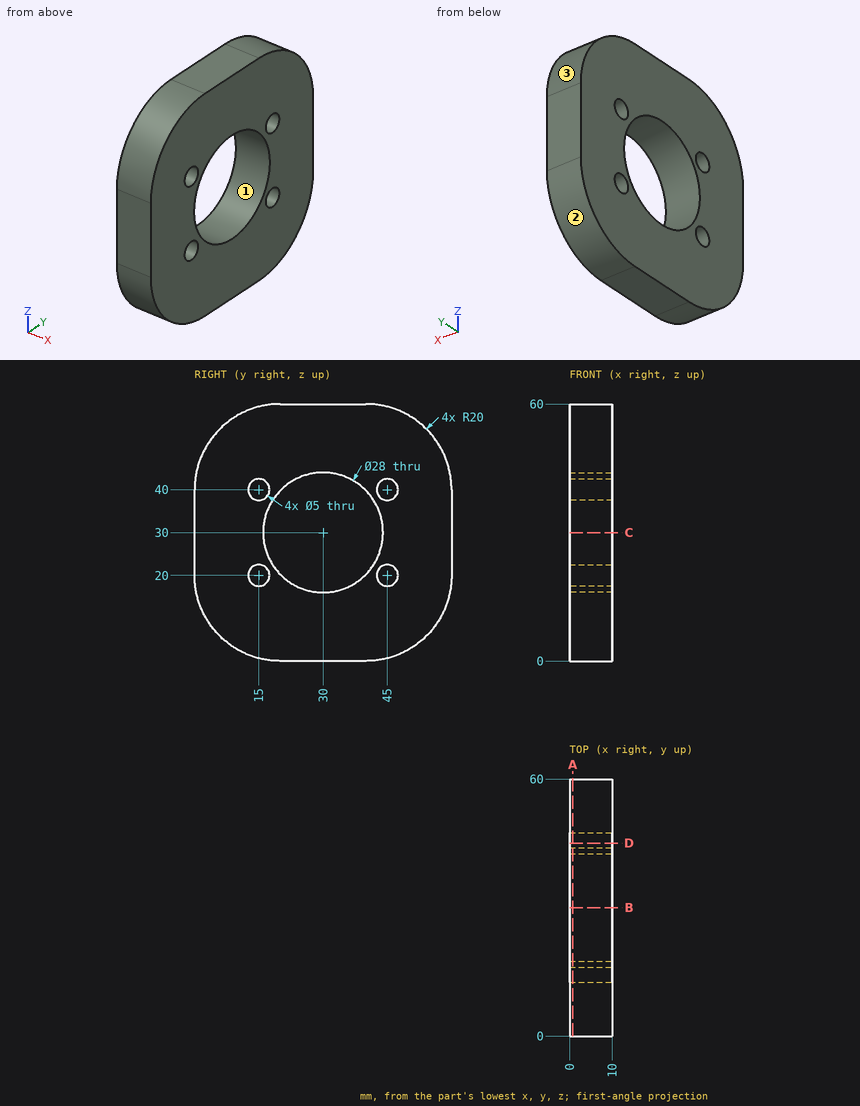
Verification items for this drawing (mm, ordinates from the low corner). Round coordinates to 2 decimals unless told otherwise and drop trailing zeros. Order: outer loops, then holes, each group sorted by start corner. A loop starts at its lowest first (then second) coordinate and runs counter-clockwise, first axis right, second up. Notation, with made-up numbers: (-30, 2) - (4, 2) arc R35 cw to (4, 41) - close; hole circle Ø6 at (2, 75). An arc over 180 degrees is marked (long way). Use CSV: the item, a comma, the result in double quotes. Start each with the question number.
1) Go/stop test with flat-tipped pins: P1, Ø2, axis at x = 6.5, z = 14, coming from the +Y side; P2, Ø1, axis at x = 4.5, y = 48.5, coming from the -Z side; P3, Ø1.5, axis at x = 7, z = 43.5, coming from the +Y side. Record where each tip stops, or that it passes through.
2) Mould release check, pull along Z, two halves, no side actions. Record for the marked faces 1, 2 and 3: +Z half, -Z half, draft (parallel to the pull), parting line (faces both ways), or undercut.
3) Section check D-D, the plane y = 45. Record the cut outline in (x, z).
4) Section check B-B, the plane y = 30. Record the cut outline in (x, z).
5) Thickness scan on L1, parallel to Y at x = 7.25, z = 30; L2, parallel to Y at x = 1, z = 41; L3, parallel to Y at x = 8, z = 20. Record the ranges inside material, lowest first.
6) Section check A-A, the plane x = 0.75. Record the cut outline in (y, z).
Answers:
1,P1,"stops at y = 59.36"
1,P2,"stops at z = 1.67"
1,P3,"stops at y = 59.81"
2,face 1,"undercut"
2,face 2,"-Z half"
2,face 3,"+Z half"
3,outline,"(0, 0.64) - (10, 0.64) - (10, 17.5) - (0, 17.5) - close; (0, 22.5) - (10, 22.5) - (10, 37.5) - (0, 37.5) - close; (0, 42.5) - (10, 42.5) - (10, 59.36) - (0, 59.36) - close"
4,outline,"(0, 0) - (10, 0) - (10, 16) - (0, 16) - close; (0, 44) - (10, 44) - (10, 60) - (0, 60) - close"
5,L1,"y = 0 to 16, 44 to 60"
5,L2,"y = 0.03 to 12.71, 17.29 to 21.34, 38.66 to 42.71, 47.29 to 59.97"
5,L3,"y = 0 to 12.5, 17.5 to 20.2, 39.8 to 42.5, 47.5 to 60"
6,outline,"(0, 20) arc R20 ccw to (20, 0) - (40, 0) arc R20 ccw to (60, 20) - (60, 40) arc R20 ccw to (40, 60) - (20, 60) arc R20 ccw to (0, 40) - close; hole circle Ø5 at (15, 20); hole circle Ø5 at (15, 40); hole circle Ø28 at (30, 30); hole circle Ø5 at (45, 20); hole circle Ø5 at (45, 40)"
